For this review, take the finished solid that the model builds, in its own axes (mm). Face numbers are marked on the shaded views. A direction names the side the tool comes from. Give positions to 0.01 mm unless a question says otherwise; leave off trailing zeros. Write each loop counter-clockwise with the first axis right and the second up, starting at its lowest first coordinate (ties: lowest second). Pieces come first, ordered by that corner, then holes.
1) Machinability: for the marked faces 4, 5, 6, 7 and 8, which of the approach directions +Z, -Z, +X, -X, +Y, -Y give a long, thin tool a straight path to every point of the face, cutting with its end or side? Answer none if there is none.
2) For P1, Ø1, axis at x = -3.5, z = 3.5, coming from the +Y side; P2, Ø10, axis at y = -7.5, z = 7.5, coming from the -X side; P3, Ø5, axis at x = -5, z = -2, coming from the -Y side; P4, Ø3, axis at x = -5.5, y = -3, coming from the +Z side, all flat-tipped, find the tip position at first contact; note any pin that passes through.
3) We need section B-B on z = 0. Give the boundary of the cut face in (x, y), and give its area (3 significant figures).
4) Draft analysis for pull direction Z (two halves, no side actions). For the marked faces 1, 2 and 3, state which applies: pulls with the +Z half, pulls with the -Z half, needs draft (parallel to the pull), parting line crosses it, or undercut.
5) We need section C-C on y = 0. Give the boundary of the cut face in (x, z), and give its area (3 significant figures).
6) We need section D-D on y = -4.5. Give the boundary of the cut face in (x, z).
7) We need section A-A on x = -5.5. Give the boundary of the cut face in (y, z), and give its area (3 significant figures).
8) Wall thickness on line 1 along Z through (x, y) = (-5, 2.75); line 2 along X through (y, z) = (-3.25, 0); line 3 along X through (y, z) = (6.75, 5.5): over which ranges is each line inside the solid? List them lowest first.
Autodesk Inventor part; units mm, degrees
ref_plane "YZ Plane" through (0, 0, 0) normal (1, 0, 0) x (0, 1, 0)
ref_plane "XZ Plane" through (0, 0, 0) normal (0, 1, 0) x (-1, 0, 0)
ref_plane "XY Plane" through (0, 0, 0) normal (0, 0, 1) x (1, 0, 0)
sketch "Sketch1" plane through (0, 0, 0) normal (1, 0, 0) x (0, 1, 0)
  circle A0 centre (0, 0) radius 10
  dimension "d0" = 20
extrude "Extrusion1" add sketch "Sketch1" along normal blind 1.5
sketch "Sketch2" plane through (0, 0, 0) normal (-1, 0, 0) x (0, 0, 1)
  line L0 (4.5, -6) -> (-4.5, -6)
  line L1 (-4.5, -6) -> (-4.5, 6)
  line L2 (-4.5, 6) -> (4.5, 6)
  line L3 (4.5, 6) -> (4.5, -6)
  line L4 (4.5, -6) -> (-4.5, 6) construction
  line L5 (-4.5, -6) -> (4.5, 6) construction
  point P0 (0, 0)
  dimension "d3" = 9
  dimension "d4" = 12
extrude "Extrusion2" add sketch "Sketch2" along normal blind 7.5
sketch "Sketch3" plane through (0, 6, 4.5) normal (0, 1, 0) x (1, 0, 0)
  line L0 (-6, 1.5) -> (0, 1.5)
  line L1 (0, 1.5) -> (0, 7.5)
  line L2 (0, 7.5) -> (-6, 7.5)
  line L3 (-6, 7.5) -> (-6, 1.5)
  line L4 (-6, 1.5) -> (0, 7.5) construction
  line L5 (0, 1.5) -> (-6, 7.5) construction
  line L6 (0, 4.5) -> (-7.5, 4.5) construction
  line L7 (-7.5, 9) -> (-7.5, 0) construction
  line L8 (0, 14.5) -> (0, -5.5) construction
  point P0 (-3, 4.5)
  point P1 (-3, 4.5)
  dimension "d7" = 0
  dimension "d8" = 6
  dimension "d9" = 6
extrude "Extrusion3" cut sketch "Sketch3" against normal through all
fillet "Fillet1" radius 2 2 edges at (0, 0, -4.5) (0, 0, 4.5)
properties part number "foot_holder"
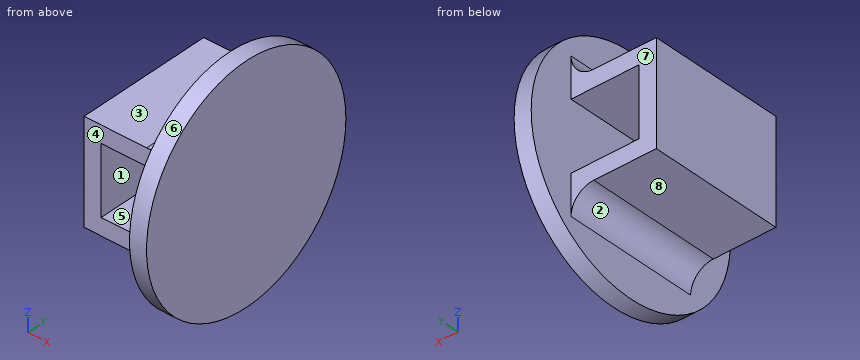
Results list:
1. face 4: +Z, -Z, -X, -Y
1. face 5: +Y, -Y
1. face 6: +X, -X
1. face 7: +Z, -Z, -X, +Y
1. face 8: -Z, -X, +Y, -Y
2. P1: stops at y = 6
2. P2: stops at x = -7.5
2. P3: stops at y = -6
2. P4: stops at z = 4.5
3. outline: (-7.5, -6) - (-6, -6) - (-6, 6) - (-7.5, 6) - close; (0, -10) - (1.5, -10) - (1.5, 10) - (0, 10) - close
3. area: 48.0 mm2
4. face 1: undercut
4. face 2: pulls with the -Z half
4. face 3: pulls with the +Z half
5. outline: (-7.5, -4.5) - (-2, -4.5) arc R2 cw to (0, -6.5) - (0, -10) - (1.5, -10) - (1.5, 10) - (0, 10) - (0, 6.5) arc R2 cw to (-2, 4.5) - (-7.5, 4.5) - close; hole (-6, -3) - (0, -3) - (0, 3) - (-6, 3) - close
5. area: 63.2 mm2
6. outline: (-7.5, -4.5) - (-2, -4.5) arc R2 cw to (0, -6.5) - (0, -8.93) - (1.5, -8.93) - (1.5, 8.93) - (0, 8.93) - (0, 6.5) arc R2 cw to (-2, 4.5) - (-7.5, 4.5) - close; hole (-6, -3) - (0, -3) - (0, 3) - (-6, 3) - close
7. outline: (-6, -4.5) - (6, -4.5) - (6, -3) - (-6, -3) - close; (-6, 3) - (6, 3) - (6, 4.5) - (-6, 4.5) - close
7. area: 36.0 mm2
8. line 1: z = -4.5 to -3, 3 to 4.5
8. line 2: x = -7.5 to -6, 0 to 1.5
8. line 3: x = 0 to 1.5
